```python
from build123d import *

# Parameters (mm, degrees)
SKETCH1_R                            = 66.675
BOSS_EXTRUDE1_DEPTH                  = 6.35
SKETCH2_R                            = 39.6875
BOSS_EXTRUDE2_DEPTH                  = 10.16
FILLET1_R                            = 2.54
SKETCH5_R                            = 23.749
CUT_EXTRUDE1_DEPTH                   = 11.557
F_1_4_0_25_DIAMETER_HOLE1_D          = 6.35
F_1_4_0_25_DIAMETER_HOLE1_DEPTH      = 6.351
CIRPATTERN1_COUNT                    = 6
SKETCH8_W                            = 5.334
SKETCH8_H                            = 2.7178
Q_0_332_DIAMETER_HOLE1_D             = 8.4328
Q_0_332_DIAMETER_HOLE1_DEPTH         = 8.89
Q_0_332_DIAMETER_HOLE1_TIP           = 2.533468714
F_3_32_0_09375_DIAMETER_HOLE1_D      = 2.38125
SKETCH16_R                           = 14.2875
BOSS_EXTRUDE3_DEPTH                  = 10.16
F_45_64_0_70313_DIAMETER_HOLE1_D     = 17.859502
F_45_64_0_70313_DIAMETER_HOLE1_DEPTH = 15.113


with BuildPart() as part:
    # Sketch1 → Boss-Extrude1 (new body)
    with BuildSketch(Plane(origin=(0, 0, 0), x_dir=(1, 0, 0), z_dir=(0, 1, 0))):
        Circle(SKETCH1_R)
    extrude(amount=BOSS_EXTRUDE1_DEPTH)

    # Sketch2 → Boss-Extrude2 (add)
    with BuildSketch(Plane(origin=(0, 6.35, 0), x_dir=(1, 0, 0), z_dir=(0, 1, 0))):
        Circle(SKETCH2_R)
    extrude(amount=BOSS_EXTRUDE2_DEPTH)

    # Fillet1
    fillet1_edges = [part.edges().sort_by_distance(p)[0] for p in [
        (-39.6875, 6.35, 0),
    ]]
    fillet(fillet1_edges, radius=FILLET1_R)

    # Sketch5 → Cut-Extrude1 (cut)
    with BuildSketch(Plane.XZ):
        Circle(SKETCH5_R)
    extrude(amount=-CUT_EXTRUDE1_DEPTH, mode=Mode.SUBTRACT)

    # 1/4 (0.25) Diameter Hole1
    with Locations(Plane(origin=(0, 6.35, 0), x_dir=(1, 0, 0), z_dir=(0, 1, 0))):
        with Locations((-57.15, 0)):
            f_1_4_0_25_diameter_hole1 = Hole(F_1_4_0_25_DIAMETER_HOLE1_D / 2, depth=F_1_4_0_25_DIAMETER_HOLE1_DEPTH)

    # CirPattern1: 1/4 (0.25) Diameter Hole1 ×6 about axis
    cirpattern1_axis = Axis((0, 0, 0), (0, 1, 0))
    for i in range(1, CIRPATTERN1_COUNT):
        add(f_1_4_0_25_diameter_hole1.rotate(cirpattern1_axis, i * 360 / CIRPATTERN1_COUNT), mode=Mode.SUBTRACT)

    # Sketch8 → Cut-Revolve1 (revolve, cut)
    with BuildSketch(Plane.XY):
        with Locations((40.2844, 1.3589)):
            Rectangle(SKETCH8_W, SKETCH8_H)
    revolve(axis=Axis((0, -1.27, 0), (0, 1, 0)), mode=Mode.SUBTRACT)

    # Q (0.332) Diameter Hole1
    with Locations(Plane(origin=(0, 16.51, 0), x_dir=(1, 0, 0), z_dir=(0, 1, 0))):
        with Locations((31.75, 0)):
            Hole(Q_0_332_DIAMETER_HOLE1_D / 2, depth=Q_0_332_DIAMETER_HOLE1_DEPTH)
            with Locations((0, 0, -(Q_0_332_DIAMETER_HOLE1_DEPTH + Q_0_332_DIAMETER_HOLE1_TIP / 2))):  # 118° drill point
                Cone(0, Q_0_332_DIAMETER_HOLE1_D / 2, Q_0_332_DIAMETER_HOLE1_TIP, mode=Mode.SUBTRACT)

    # 3/32 (0.09375) Diameter Hole1 (through all)
    with Locations(Plane(origin=(0, 0, 0), x_dir=(-1, 0, 0), z_dir=(0, -1, 0))):
        with Locations((-31.75, 0)):
            Hole(F_3_32_0_09375_DIAMETER_HOLE1_D / 2)

    # Sketch16 → Boss-Extrude3 (add)
    with BuildSketch(Plane(origin=(0, 16.51, 0), x_dir=(1, 0, 0), z_dir=(0, 1, 0))):
        Circle(SKETCH16_R)
    extrude(amount=BOSS_EXTRUDE3_DEPTH)

    # 45/64 (0.70313) Diameter Hole1
    with Locations(Plane(origin=(0, 26.67, 0), x_dir=(1, 0, 0), z_dir=(0, 1, 0))):
        with Locations((0, 0)):
            Hole(F_45_64_0_70313_DIAMETER_HOLE1_D / 2, depth=F_45_64_0_70313_DIAMETER_HOLE1_DEPTH)


solid = part.part
```
Source: CAD feature listing. Evaluate the final solid. Frame: model axes, mm. A direction names the side the tool comes from. Round coordinates to 2 decimals unless told otherwise and drop trailing zeros. Loops run counter-clockwise (first coordinate to the right, second up) from the corner with the lowest first, then second, coordinate; pieces in that order, holes last.
1. Ray query, L1, parallel to Z at x = 0, y = 1.25 (3 decimals); L2, parallel to X at y = 8.25, z = 3.5; L3, parallel to Z at x = 0.5, y = 21.75. Return the intervals inside material, ascending.
2. Contact query for flat-ended pins moving along their axis: pin 1 (8 mm diameter, centred on x = -29, y = 17, fed in from +Z); pin 2 (10 mm diameter, centred on x = -28.58, z = -49.49, fed in from +Y); pin 3 (1 mm diameter, centred on y = 5, z = -39, fed in from -X). Output: stop coordinate, or through.
3. Section query D-D on z = -59. Output: boundary loops of the cut face in (x, y).
4. Section query B-B on x = 57.15. Output: boundary loops of the cut face in (y, z) (3 decimals), and give its area (3 significant figures).
5. Access query for faces 1 (the cylindrical face through (37.855, 12.647, -11.921)), 2 (the cylindrical face through (-9.31, 1.38, 41.93)), 3 (the cylindrical face through (-53.98, 3.13, -0.14)). Directions: +Z, -Z, +X, -X, +Y, -Y. A direction counts if a zero-diameter tool reaches every point of the face in a straight line with its end or side. Return the directions, or none.
6. Section query C-C on z = 57. Output: boundary loops of the cut face in (x, y).
7. Mould query, pull axis Z, two halves, no side actions, for faces 4 (the cylindrical face through (-14.274, 21.519, -0.628)), 5 (the flat face through (-1, 0, 44)), 6 (the cylindrical face through (-8.155, 1.378, 36.723)). Classes: released by +Z, released by -Z, zero draft, split by the parting line, or undercut.
Answers below:
1. L1: z = -66.675 to -42.951, -37.617 to -23.749, 23.749 to 37.617, 42.951 to 66.675
1. L2: x = -39.62 to -23.49, 23.49 to 29.4, 34.1 to 39.62
1. L3: z = -14.28 to -8.92, 8.92 to 14.28
2. pin 1: stops at z = 30.8
2. pin 2: stops at y = 6.35
2. pin 3: stops at x = -54.44
3. outline: (-31.06, 0) - (31.06, 0) - (31.06, 6.35) - (-31.06, 6.35) - close
4. outline: (0, -34.343) - (6.35, -34.343) - (6.35, -3.175) - (0, -3.175) - close; (0, 3.175) - (6.35, 3.175) - (6.35, 34.343) - (0, 34.343) - close
4. area: 396 mm2
5. face 1: +Y
5. face 2: -Y
5. face 3: +Y, -Y
6. outline: (-34.59, 0) - (34.59, 0) - (34.59, 6.35) - (-34.59, 6.35) - close
7. face 4: split by the parting line
7. face 5: zero draft
7. face 6: undercut
